Geometry: final body of the model. Coordinates: model frame, mm. Give positions to 0.01 mm unless a question says otherwise; leave off trailing zeros. Write each loop counter-clockwise with the first axis right and the second up, starting at its lowest first coordinate (ties: lowest second). Pieces come first, ordered by that corner, then holes.
Q1. Section C-C (z = 164). Return the cut outline in (x, y) (3 decimals), plus the area to 3 significant figures.
Q2. Line query: line 1 (Z direction, x = 17.25, y = 0); line 2 (X direction, y = 7.5, z = 209.5) (3 decimals). Output: solid intervals per line, ascending.
Q3. Section B-B (y = 0). State how many separate pieces and enclosed holes the cut face has, plus the area to 3 significant figures.
Q4. Pin query (flat end, axial travel): pin 1 Ø4 at (x, z) = (0, 287.5) entering from +Y. Return the tip coordinate at first contact, or that it passes through.
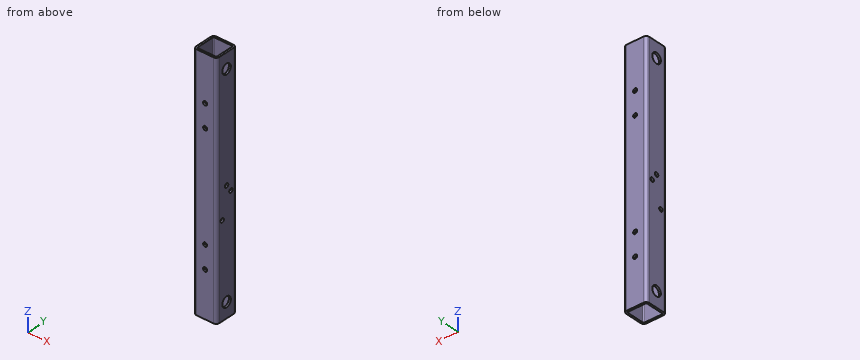
from build123d import *

# Parameters (mm, degrees)
BOSS_EXTRUDE1_DEPTH             = 400
CUT_EXTRUDE1_DEPTH              = 401.906229685
CUT_EXTRUDE1_DEPTH_BACK         = 401.906229685
SKETCH2_R                       = 8.3125
CUT_EXTRUDE2_DEPTH              = 401.906229685
CUT_EXTRUDE2_DEPTH_BACK         = 401.906229685
SKETCH3_R                       = 3.38
CUT_EXTRUDE3_DEPTH              = 401.906229685
CUT_EXTRUDE3_DEPTH_BACK         = 401.906229685
SKETCH4_R                       = 3.38
CUT_EXTRUDE4_DEPTH              = 401.906229685
CUT_EXTRUDE4_DEPTH_BACK         = 401.906229685
SKETCH5_R                       = 3.38
BROOM_MOUNTING_HOLES_DEPTH      = 401.906229685
BROOM_MOUNTING_HOLES_DEPTH_BACK = 401.906229685
SKETCH6_R                       = 3.38


with BuildPart() as part:
    # Sketch1 → Boss-Extrude1 (new body)
    with BuildSketch(Plane.XY):
        with BuildLine():
            Line((-14.05, 19.05), (14.05, 19.05))
            ThreePointArc((14.05, 19.05), (17.585533906, 17.585533906), (19.05, 14.05))
            Line((19.05, 14.05), (19.05, -14.05))
            ThreePointArc((19.05, -14.05), (17.585533906, -17.585533906), (14.05, -19.05))
            Line((14.05, -19.05), (-14.05, -19.05))
            ThreePointArc((-14.05, -19.05), (-17.585533906, -17.585533906), (-19.05, -14.05))
            Line((-19.05, -14.05), (-19.05, 14.05))
            ThreePointArc((-19.05, 14.05), (-17.585533906, 17.585533906), (-14.05, 19.05))
        make_face()
        with BuildLine():
            Line((-15.875, 14.05), (-15.875, -14.05))
            ThreePointArc((-15.875, -14.05), (-15.340469876, -15.340469876), (-14.05, -15.875))
            Line((-14.05, -15.875), (14.05, -15.875))
            ThreePointArc((14.05, -15.875), (15.340469876, -15.340469876), (15.875, -14.05))
            Line((15.875, -14.05), (15.875, 14.05))
            ThreePointArc((15.875, 14.05), (15.340469876, 15.340469876), (14.05, 15.875))
            Line((14.05, 15.875), (-14.05, 15.875))
            ThreePointArc((-14.05, 15.875), (-15.340469876, 15.340469876), (-15.875, 14.05))
        make_face(mode=Mode.SUBTRACT)
    extrude(amount=BOSS_EXTRUDE1_DEPTH)

    # Sketch2 → Cut-Extrude1 (cut, two sides: drawn at the far end of the back side and taken through both)
    with BuildSketch(Plane(origin=(0, 0, 0), x_dir=(0, 0, -1), z_dir=(1, 0, 0)).offset(-CUT_EXTRUDE1_DEPTH_BACK)):
        with Locations((-375, 0)):
            Circle(SKETCH2_R)
        with Locations((-25, 0)):
            Circle(SKETCH2_R)
    extrude(amount=CUT_EXTRUDE1_DEPTH + CUT_EXTRUDE1_DEPTH_BACK, mode=Mode.SUBTRACT)

    # Sketch3 → Cut-Extrude2 (cut, two sides: drawn at the far end of the back side and taken through both)
    with BuildSketch(Plane(origin=(0, 0, 0), x_dir=(1, 0, 0), z_dir=(0, 1, 0)).offset(-CUT_EXTRUDE2_DEPTH_BACK)):
        with Locations(Location((0, -325, 0), (0, 0, 90))):
            Circle(SKETCH3_R)
        with Locations(Location((0, -75, 0), (0, 0, 90))):
            Circle(SKETCH3_R)
    extrude(amount=CUT_EXTRUDE2_DEPTH + CUT_EXTRUDE2_DEPTH_BACK, mode=Mode.SUBTRACT)

    # Sketch4 → Cut-Extrude3 (cut, two sides: drawn at the far end of the back side and taken through both)
    with BuildSketch(Plane(origin=(0, 0, 0), x_dir=(0, 0, -1), z_dir=(1, 0, 0)).offset(-CUT_EXTRUDE3_DEPTH_BACK)):
        with Locations((-200, 0)):
            Circle(SKETCH4_R)
    extrude(amount=CUT_EXTRUDE3_DEPTH + CUT_EXTRUDE3_DEPTH_BACK, mode=Mode.SUBTRACT)

    # Sketch5 → Cut-Extrude4 (cut, two sides: drawn at the far end of the back side and taken through both)
    with BuildSketch(Plane(origin=(0, 0, 0), x_dir=(0, 0, -1), z_dir=(1, 0, 0)).offset(-CUT_EXTRUDE4_DEPTH_BACK)):
        with Locations((-188.126155741, 8.452365235)):
            Circle(SKETCH5_R)
        with Locations((-151.873844259, -8.452365235)):
            Circle(SKETCH5_R)
    extrude(amount=CUT_EXTRUDE4_DEPTH + CUT_EXTRUDE4_DEPTH_BACK, mode=Mode.SUBTRACT)

    # Sketch6 → Broom Mounting Holes (cut, two sides: drawn at the far end of the back side and taken through both)
    with BuildSketch(Plane(origin=(0, 0, 0), x_dir=(1, 0, 0), z_dir=(0, 1, 0)).offset(-BROOM_MOUNTING_HOLES_DEPTH_BACK)):
        with Locations(Location((0, -112.5, 0), (0, 0, 270))):
            Circle(SKETCH6_R)
        with Locations(Location((0, -287.5, 0), (0, 0, 270))):
            Circle(SKETCH6_R)
    extrude(amount=BROOM_MOUNTING_HOLES_DEPTH + BROOM_MOUNTING_HOLES_DEPTH_BACK, mode=Mode.SUBTRACT)


solid = part.part
Computed:
1. outline: (-19.05, -14.05) arc R5 ccw to (-14.05, -19.05) - (14.05, -19.05) arc R5 ccw to (19.05, -14.05) - (19.05, 14.05) arc R5 ccw to (14.05, 19.05) - (-14.05, 19.05) arc R5 ccw to (-19.05, 14.05) - close; hole (-15.875, -14.05) arc R1.825 ccw to (-14.05, -15.875) - (14.05, -15.875) arc R1.825 ccw to (15.875, -14.05) - (15.875, 14.05) arc R1.825 ccw to (14.05, 15.875) - (-14.05, 15.875) arc R1.825 ccw to (-15.875, 14.05) - close
1. area: 425 mm2
2. line 1: z = 0 to 16.69, 33.31 to 196.62, 203.38 to 366.69, 383.31 to 400
2. line 2: x = -19.05 to -15.875, 15.875 to 19.05
3. separate pieces: 8
3. enclosed holes: 0
3. area: 2,290 mm2
4. pin 1: passes through
